Work out the finished part from the listing and answer in its coordinate system (mm). Face numbers are marked on the shaded views. A direction names the side the tool comes from. Give positions to 0.01 mm unless a question says otherwise; leave off trailing zeros. Order: outer loops, then holes, each group sorted by start corner. A loop starts at its lowest first (then second) coordinate and runs counter-clockwise, first axis right, second up. Notation, with made-up numbers: (27.5, 13.25) - (80.5, 13.25) arc R22 ccw to (80.5, 32.25) - close; hole circle Ø8 at (33.25, 82.25). An arc over 180 degrees is marked (long way). Return JSON: item names as keys, results as strings. Group by question number.
Autodesk Inventor part; units mm, degrees
ref_plane "YZ Plane" through (0, 0, 0) normal (1, 0, 0) x (0, 1, 0)
ref_plane "XZ Plane" through (0, 0, 0) normal (0, 1, 0) x (-1, 0, 0)
ref_plane "XY Plane" through (0, 0, 0) normal (0, 0, 1) x (1, 0, 0)
sketch "Sketch1" plane through (0, 0, 0) normal (0, 0, 1) x (1, 0, 0)
  line L0 (0, 25.4) -> (0, 0)
  line L1 (0, 0) -> (25.4, 0)
  line L2 (25.4, 0) -> (25.4, 3.175)
  line L3 (25.4, 3.175) -> (3.175, 3.175)
  line L4 (3.175, 3.175) -> (3.175, 25.4)
  line L5 (3.175, 25.4) -> (0, 25.4)
  dimension "d0" = 3.175
  dimension "d1" = 3.175
  dimension "d2" = 25.4
  dimension "d3" = 25.4
extrude "Extrusion1" add sketch "Sketch1" along normal blind 76.2
fillet "Fillet1" radius 3.175 4 edges at (1.5875, 25.4, 76.2) (1.5875, 25.4, 0) (25.4, 1.5875, 0) (25.4, 1.5875, 76.2)
sketch "Sketch2" plane through (0, 0, 0) normal (-1, 0, 0) x (0, 0, 1)
  line L0 (0, 0) -> (76.2, 0)
  line L1 (3.175, 25.4) -> (73.025, 25.4)
  circle A0 centre (38.1, 12.7) radius 4.7625
  line L2 (38.1, 25.4) -> (38.1, 12.7)
  line L3 (38.1, 12.7) -> (38.1, 0)
  dimension "d7" = 9.525
extrude "Extrusion2" cut sketch "Sketch2" against normal up to next
sketch "Sketch3" plane through (0, 0, 0) normal (0, -1, 0) x (1, 0, 0)
  line L0 (22.225, 76.2) -> (0, 76.2)
  line L1 (0, 0) -> (0, 76.2)
  line L2 (22.225, 0) -> (0, 0)
  line L3 (25.4, 3.175) -> (25.4, 73.025)
  line L4 (0, 63.5) -> (12.7, 63.5)
  line L5 (12.7, 63.5) -> (25.4, 63.5)
  line L6 (12.7, 76.2) -> (12.7, 63.5)
  line L7 (12.7, 63.5) -> (12.7, 12.7)
  line L8 (12.7, 12.7) -> (12.7, 0)
  circle A0 centre (12.7, 63.5) radius 3.175
  circle A1 centre (12.7, 12.7) radius 3.175
  dimension "d10" = 12.7
  dimension "d11" = 6.35
  dimension "d12" = 6.35
extrude "Extrusion3" cut sketch "Sketch3" against normal up to next contours A0 L5 L6 | L6 L4 A0 | L7 A0 L4 | L5 A0 L7 | A1 L8 L7 | L7 L8 A1
properties part number "WheelBlockMount" material "Aluminum-6061"
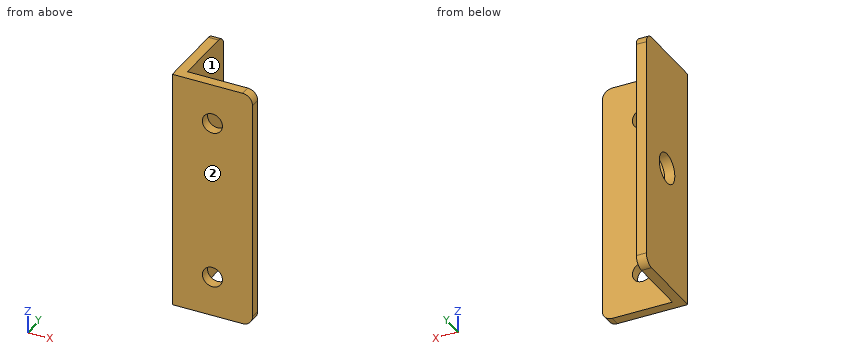
1. The part is cut by section A-A (z = 38.1). Give the vertices of the cut face in (x, y) (1 decimal).
2. The part is cut by section D-D (z = 20.5). Give the vertices of the cut face in (x, y) (3 decimals), and give its area (3 significant figures).
3. The part is cut by section B-B (x = 12.7). Give the vertices of the cut face in (y, z) (3 decimals), and give its area (3 significant figures).
4. A tool of negligible diameter and unlimited length cuts with its end or side. For the marked faces 1 and 2, from which of +Z, -Z, +X, -X, +Y, -Y can it reach the whole face along a straight path? Write none if from no direction.
5. Consider probe 1 along Z at (x, y) = (12.7, 1.2) (3 decimals); probe 2 along Z at (x, y) = (0.8, 12.7); probe 3 along X at (y, z) = (0.95, 12.7) (3 decimals). Determine where each line is inside the solid, lowest interval first. Write a range as from..to.
6. The part is cut by section C-C (y = 12.7). Give the vertices of the cut face in (x, z) (1 decimal).
7. Each of these flat-tipped pins is pushed along its axis until it touches: pin 1 (4 mm diameter, centred on x = 12.7, z = 63.5, fed in from -Y); pin 2 (3 mm diameter, centred on y = 19.5, z = 17.5, fed in from +X) (3 decimals). Where does it stop, or does it pass through?
Answers:
{
 "1": {"outline": "(0, 0) - (25.4, 0) - (25.4, 3.2) - (3.2, 3.2) - (3.2, 7.9) - (0, 7.9) - close; (0, 17.5) - (3.2, 17.5) - (3.2, 25.4) - (0, 25.4) - close"},
 "2": {"outline": "(0, 0) - (25.4, 0) - (25.4, 3.175) - (3.175, 3.175) - (3.175, 25.4) - (0, 25.4) - close", "area": "151 mm^2"},
 "3": {"outline": "(0, 0) - (3.175, 0) - (3.175, 9.525) - (0, 9.525) - close; (0, 15.875) - (3.175, 15.875) - (3.175, 60.325) - (0, 60.325) - close; (0, 66.675) - (3.175, 66.675) - (3.175, 76.2) - (0, 76.2) - close", "area": "202 mm^2"},
 "4": {"face 1": "+Z, -Z, +X, +Y", "face 2": "+Z, -Z, +X, -X, -Y"},
 "5": {"probe 1": "z = 0..9.525, 15.875..60.325, 66.675..76.2", "probe 2": "z = 0..33.34, 42.86..76.2", "probe 3": "x = 0..9.525, 15.875..25.4"},
 "6": {"outline": "(0, 0) - (3.2, 0) - (3.2, 33.3) - (0, 33.3) - close; (0, 42.9) - (3.2, 42.9) - (3.2, 76.2) - (0, 76.2) - close"},
 "7": {"pin 1": "passes through", "pin 2": "stops at x = 3.175"}
}
